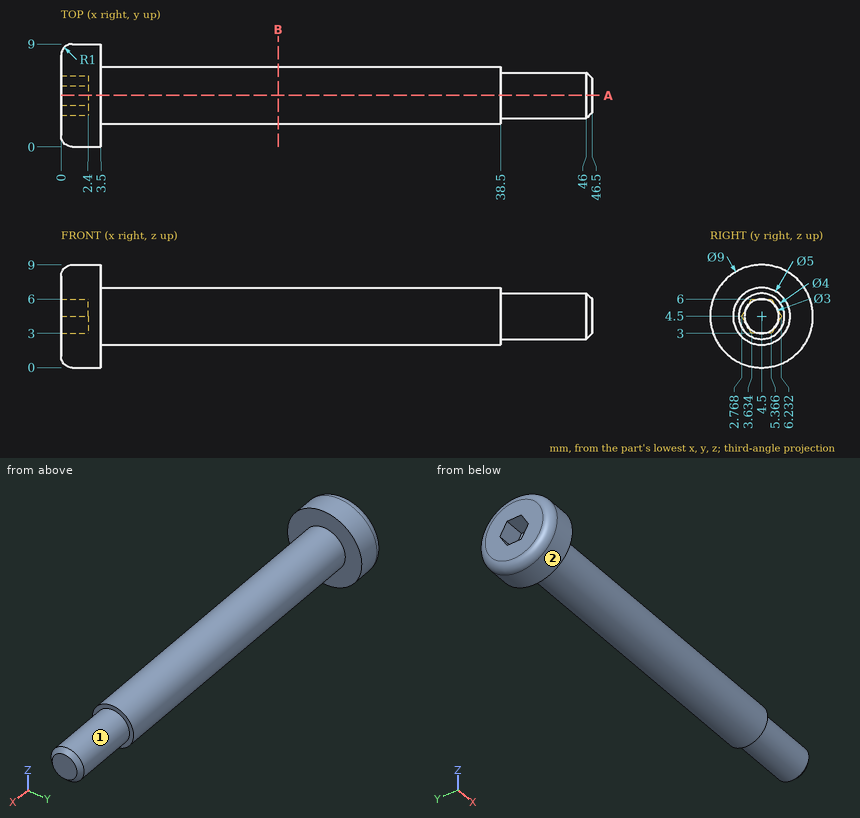
Study the drawing (mm; zero at the part's minimum x, y, z) and answer. A direction names the side the tool comes from. Coordinates: 2 decimals unless noted, no trailing zeros. Write each loop counter-clockwise with the first axis right and the second up, starting at its lowest first coordinate (ties: lowest second). Pieces come first, ordered by that corner, then holes.
Q1. Which of the six approach directions +Z, -Z, +X, -X, +Y, -Y give full straight-line access (tool end or side, diameter ignored) to the marked faces 1 and 2?
Q2. Find the intervals of material crossed by line 1 (X direction, y = 3, z = 3); line 2 (Z direction, x = 6, y = 2.5); line 3 (Y direction, x = 31.5, z = 4.5), in increasing order.
Q3. Each of these flat-tipped pins is pushed along its axis until it touches: pin 1 Ø2 at (x, y) = (25, 4.5) entering from +Z; pin 2 Ø3 at (x, y) = (41.5, 5.5) entering from +Z; pin 3 Ø3 at (y, z) = (1.5, 1.5) entering from +X. Where does it stop, or does it pass through?
Q4. A cutting plane is placed at A-A, the plane y = 4.5. Give the vertices of the cut face in (x, z), then the cut area to 3 significant figures.
Q5. A cutting plane is placed at B-B, the plane x = 19. Give the vertices of the cut face in (y, z).
Findings below:
1. face 1: +X
1. face 2: +X, -X
2. line 1: x = 0 to 38.5
2. line 2: z = 3 to 6
2. line 3: y = 2 to 7
3. pin 1: stops at z = 7
3. pin 2: stops at z = 6.5
3. pin 3: stops at x = 3.5
4. outline: (0, 1) arc R1 ccw to (1, 0) - (3.5, 0) - (3.5, 2) - (38.5, 2) - (38.5, 2.5) - (46, 2.5) - (46.5, 3) - (46.5, 6) - (46, 6.5) - (38.5, 6.5) - (38.5, 7) - (3.5, 7) - (3.5, 9) - (1, 9) arc R1 ccw to (0, 8) - (0, 6) - (2.4, 6) - (2.4, 3) - (0, 3) - close
4. area: 231 mm2
5. outline: circle Ø5 at (4.5, 4.5)
